from build123d import *

# Parameters (mm, degrees)
F2_W     = 20
F2_H     = 100
F3_DEPTH = 35
F4_W     = 20
F4_H     = 20
F5_DEPTH = 20


with BuildPart() as f1:
    # F0 (on Front) → F1 (revolve)
    with BuildSketch(Plane.XZ):
        Polygon((-108.390996, 30), (-138.390996, 30), (-138.390996, 12.5), (-178.390996, 12.5), (-178.390996, 0), (155.390996, 0), (155.390996, 30), (150.890996, 25), (147.890996, 25), (143.390996, 30), (143.390996, 12.5), (138.390996, 12.5), (138.390996, 30), (108.390996, 30), (100, 20), (-100, 20), align=None)
    revolve(axis=Axis((-3.867105, 0, 0), (1, 0, 0)))

    # F2 (on Top) → F3 (join)
    with BuildSketch(Plane.XY):
        with Locations((-125, 0)):
            Rectangle(F2_W, F2_H)
        with Locations((125, 0)):
            Rectangle(F2_W, F2_H)
    extrude(amount=-F3_DEPTH)

    # F4 (on face) → F5 (cut)
    with BuildSketch(Plane.XY):
        with Locations((-125, 40)):
            Rectangle(F4_W, F4_H)
        with Locations((-125, -40)):
            Rectangle(F4_W, F4_H)
        with Locations((125, -40)):
            Rectangle(F4_W, F4_H)
        with Locations((125, 40)):
            Rectangle(F4_W, F4_H)
    extrude(amount=-F5_DEPTH, mode=Mode.SUBTRACT)


solid = f1.part
The listing builds one solid part. Answer for the finished solid, in the listing's coordinates (mm). A direction names the side the tool comes from. Coordinates: 2 decimals unless noted, no trailing zeros. Loops run counter-clockwise (first coordinate to the right, second up) from the corner with the lowest first, then second, coordinate; pieces in that order, holes last. Notation, with made-up numbers: M 66,39 L 114,39 A21 ccw 114,67 Z; hole C 26.5,-5 d6. An arc over 180 degrees is marked long. Answer in a Markdown table with one row per item.
1) Find section B-B (x = 12). Determine the outline of the cut face in (y, z), then the cut area to 3 significant figures.
Answers below:
| item | result |
|---|---|
| outline | C 0,0 d40 |
| area | 1,260 mm^2 |
2) Find the intervals of material crossed by probe 1 along X at (y, z) = (-7, 14); probe 2 along X at (y, z) = (-5.5, 20); probe 3 along X at (y, z) = (23, 17.5), in increasing order.
Answers below:
| item | result |
|---|---|
| probe 1 | -138.39 to 138.39, 143.39 to 155.39 |
| probe 2 | -138.39 to -100.62, 100.62 to 138.39, 143.39 to 155.39 |
| probe 3 | -138.39 to -107.47, 107.47 to 138.39, 143.39 to 144.38, 154.4 to 155.39 |
3) Find section C-C (x = -148). Determine the outline of the cut face in (y, z).
Answers below:
| item | result |
|---|---|
| outline | C 0,0 d25 |
4) Which of the six approach directions +Z, -Z, +X, -X, +Y, -Y give full straight-line access (tool end or side, diameter ignored) to faces 5 (the flat face through (-115, -4, -30)), 6 (the cylindrical face through (-158.671, -3.755, 11.923)), 7 (the cylindrical face through (123.181, -9.011, 28.615))?
Answers below:
| item | result |
|---|---|
| face 5 | -Z |
| face 6 | -X |
| face 7 | none |
5) Given pin 1 (10.5 mm diameter, centred on y = 5.5, z = -25.5, fed in from -X); pin 2 (16 mm diameter, centred on x = 127, z = -9, fed in from -Y); pin 3 (10 mm diameter, centred on x = -129.5, y = -38, fed in from +Z); pin 4 (3 mm diameter, centred on x = 67.5, y = -23, fed in from -Z), each flat-ended and moving along its own axis, determine where each tip first touches the part or whether it passes through.
Answers below:
| item | result |
|---|---|
| pin 1 | x = -138.39 |
| pin 2 | y = -30 |
| pin 3 | z = -20 |
| pin 4 | through |
6) Determine the mould class of faces 1 (the flat face through (155.391, 0, 0)), 2 (the cylindrical face through (149.37, -7.509, 23.846)), 3 (the flat face through (-125, 1, -35)), 4 (the flat face through (-138.391, 13, 0)) for opening direction X: released by +X, released by -X, zero draft, split by the parting line, or undercut.
Answers below:
| item | result |
|---|---|
| face 1 | released by +X |
| face 2 | undercut |
| face 3 | zero draft |
| face 4 | released by -X |
7) Find section A-A (x = 123). Determine the outline of the cut face in (y, z).
Answers below:
| item | result |
|---|---|
| outline | M -50,-35 L 50,-35 L 50,-20 L 30,-20 L 30,0 A30 ccw -30,0 L -30,-20 L -50,-20 Z |
